For this review, take the finished solid that the model builds, in its own axes (mm). A direction names the side the tool comes from. Round coordinates to 2 decimals unless told otherwise and drop trailing zeros. Loops run counter-clockwise (first coordinate to the right, second up) from the corner with the lowest first, then second, coordinate; pieces in that order, holes last.
1) Take a section at C-C (x = 8). State the section outline as (y, z) points, then the cut area to 3 significant figures.
2) Take a section at A-A (y = 18). State the section outline as (x, z) points (3 decimals), then the cut area to 3 significant figures.
3) Take a section at B-B (z = -27.5). State the section outline as (x, y) points (3 decimals), then the cut area to 3 significant figures.
4) Tool access review of faces 1 (the flat face through (7, 0, -12.7)), 2 (the flat face through (-5.697, 18.997, -32.751)), 3 (the flat face through (0, 19, -53.213)), 4 (the flat face through (-4.41, 19, -50.71)): name each direction out of +Z, -Z, +X, -X, +Y, -Y from which nothing blocks a thin tool from reaching the whole face with its end or side.
5) Insertion check: pin 1 (3 mm diameter, centred on y = 3.5, z = -44.5, fed in from +X); pin 2 (6 mm diameter, centred on x = -4.5, z = -11.5, fed in from +Y); pin 3 (6 mm diameter, centred on x = -0.5, y = 18.5, fed in from +Z). Each pin has a flat end and moves straight along its axis. Give the tip position at first contact, or say it passes through.
6) Mouldability with a two-part tool opening along Z and no side actions: class faces 5 (the conical face through (-2.525, -1.936, -73.498)), 6 (the flat face through (-1, -9, -23.368)), 7 (the flat face through (3, -3, -65.278)) as pulls with the +Z half, pulls with the -Z half, needs draft (parallel to the pull), parting line crosses it, or undercut.
7) Wall thickness on L1, parallel to Y at x = 0, z = -24 (3 decimals); L2, parallel to X at y = 0, z = -33 (3 decimals); L3, parallel to Y at x = 0, z = -13.5 (3 decimals): over which ranges is each line inside the solid? List them lowest first.
8) Take a section at D-D (y = -5.5). State the section outline as (x, z) points, then the cut area to 3 significant figures.
```python
from build123d import *
from OCP.BRepFilletAPI import BRepFilletAPI_MakeChamfer

# Parameters (mm, degrees)
SKETCH3_R           = 10.16
CUT_EXTRUDE1_DEPTH  = 10.668
SKETCH4_R           = 6.985
BOSS_EXTRUDE1_DEPTH = 5.08
SKETCH5_W           = 13.97
SKETCH5_H           = 30.48
BOSS_EXTRUDE2_DEPTH = 7.62
CHAMFER1_SIZE       = 5.08
CHAMFER2_SIZE       = 20.32
CHAMFER2_SIZE2      = 2.54


# Read off the part's stored shape, not the designer's step: LPattern8
with BuildPart() as part:
    # Sketch1 → Revolve1 (revolve)
    with BuildSketch(Plane(origin=(0, 0, 0), x_dir=(1, 0, 0), z_dir=(0, 1, 0))):
        Polygon((3.81, 85.598), (3.81, 65.278), (11.684, 65.278), (11.684, 23.368), (10.16, 23.368), (10.16, 12.7), (6.35, 12.7), (6.35, 0), (3.175, 0), (3.175, 65.278), (1.905, 85.598), align=None)
    revolve(axis=Axis((0, 0, 0), (0, 0, -1)))

    # Sketch2 → Cut-Revolve1 (revolve, cut)
    with BuildSketch(Plane(origin=(0, 0, 0), x_dir=(1, 0, 0), z_dir=(0, 1, 0))):
        Polygon((3.81, 85.598), (2.794, 85.598), (3.81, 80.518), align=None)
    revolve(axis=Axis((0, 0, 0), (0, 0, 1)), mode=Mode.SUBTRACT)

    # LPattern8 outline → LPattern8 (revolve, cut)
    with BuildSketch(Plane.XZ):
        Polygon((3.81, -75.438), (2.794, -80.518), (3.81, -80.518), align=None)
        Polygon((2.794, -75.438), (3.81, -75.438), (3.81, -70.358), align=None)
    revolve(axis=Axis((0, 0, 0), (0, 0, 1)), mode=Mode.SUBTRACT)

    # Sketch3 → Cut-Extrude1 (cut)
    with BuildSketch(Plane.XY.offset(-12.7)):
        Circle(SKETCH3_R)
        Polygon((5.0165, -8.688832876), (10.033, 0), (5.0165, 8.688832876), (-5.0165, 8.688832876), (-10.033, 0), (-5.0165, -8.688832876), align=None, mode=Mode.SUBTRACT)
    extrude(amount=-CUT_EXTRUDE1_DEPTH, mode=Mode.SUBTRACT)

    # Sketch4 → Boss-Extrude1 (add)
    with BuildSketch(Plane(origin=(0, 10.16, 0), x_dir=(1, 0, 0), z_dir=(0, 1, 0))):
        with Locations(Location((0, 44.323, 0), (0, 0, 34.307651456))):
            Circle(SKETCH4_R)
    extrude(amount=BOSS_EXTRUDE1_DEPTH)

    # Sketch5 → Boss-Extrude2 (add)
    with BuildSketch(Plane(origin=(0, 15.24, 0), x_dir=(1, 0, 0), z_dir=(0, 1, 0))):
        with Locations((0, 37.973)):
            Rectangle(SKETCH5_W, SKETCH5_H)
    extrude(amount=BOSS_EXTRUDE2_DEPTH)

    # Chamfer1
    chamfer1_edges = [part.edges().sort_by_distance(p)[0] for p in [
        (-6.985, 19.05, -53.213),
        (6.985, 19.05, -53.213),
    ]]
    chamfer(chamfer1_edges, length=CHAMFER1_SIZE)

    # Chamfer2: one chamfer whose edges measure the first distance from different faces: ONE call of the kernel's chamfer builder (chamfer() names one face for all edges)
    chamfer2_edges_1 = [part.edges().sort_by_distance(p)[0] for p in [
        (-6.985, 19.05, -22.733),
    ]]
    chamfer2_side_1 = [part.faces().sort_by_distance(p)[0] for p in [
        (-6.985, 19.05, -35.433),
    ]]
    chamfer2_edges_2 = [part.edges().sort_by_distance(p)[0] for p in [
        (6.985, 19.05, -22.733),
    ]]
    chamfer2_side_2 = [part.faces().sort_by_distance(p)[0] for p in [
        (6.985, 19.05, -35.433),
    ]]
    chamfer2 = BRepFilletAPI_MakeChamfer(part.part.solid().wrapped)
    for e in chamfer2_edges_1:
        chamfer2.Add(CHAMFER2_SIZE, CHAMFER2_SIZE2, e.wrapped, chamfer2_side_1[0].wrapped)  # the first distance lies on this face
    for e in chamfer2_edges_2:
        chamfer2.Add(CHAMFER2_SIZE, CHAMFER2_SIZE2, e.wrapped, chamfer2_side_2[0].wrapped)  # the first distance lies on this face
    add(Compound.cast(chamfer2.Shape()), mode=Mode.REPLACE)


solid = part.part
```
Response:
1. outline: (-8.52, -65.28) - (8.52, -65.28) - (8.52, -23.37) - (3.52, -23.37) - (3.52, -12.7) - (-3.52, -12.7) - (-3.52, -23.37) - (-8.52, -23.37) - close
1. area: 789 mm2
2. outline: (-6.985, -48.133) - (-1.905, -53.213) - (1.905, -53.213) - (6.985, -48.133) - (6.985, -43.053) - (4.445, -22.733) - (-4.445, -22.733) - (-6.985, -43.053) - close
2. area: 348 mm2
3. outline: circle Ø23.368 at (0, 0); (-5.041, 15.24) - (5.041, 15.24) - (5.041, 22.86) - (-5.041, 22.86) - close; hole circle Ø6.35 at (0, 0)
3. area: 474 mm2
4. face 1: +Z
4. face 2: +Z, -X, +Y
4. face 3: -Z, +X, -X, +Y
4. face 4: -Z, -X, +Y
5. pin 1: stops at x = 11.51
5. pin 2: stops at y = 8.69
5. pin 3: stops at z = -22.73
6. face 5: undercut
6. face 6: pulls with the +Z half
6. face 7: pulls with the -Z half
7. L1: y = -11.684 to -3.175, 3.175 to 11.684, 15.24 to 22.86
7. L2: x = -11.684 to -3.175, 3.175 to 11.684
7. L3: y = -8.689 to -3.175, 3.175 to 8.689
8. outline: (-10.31, -65.28) - (10.31, -65.28) - (10.31, -23.37) - (6.86, -23.37) - (6.86, -12.7) - (3.17, -12.7) - (3.17, 0) - (-3.17, 0) - (-3.17, -12.7) - (-6.86, -12.7) - (-6.86, -23.37) - (-10.31, -23.37) - close
8. area: 1,090 mm2
